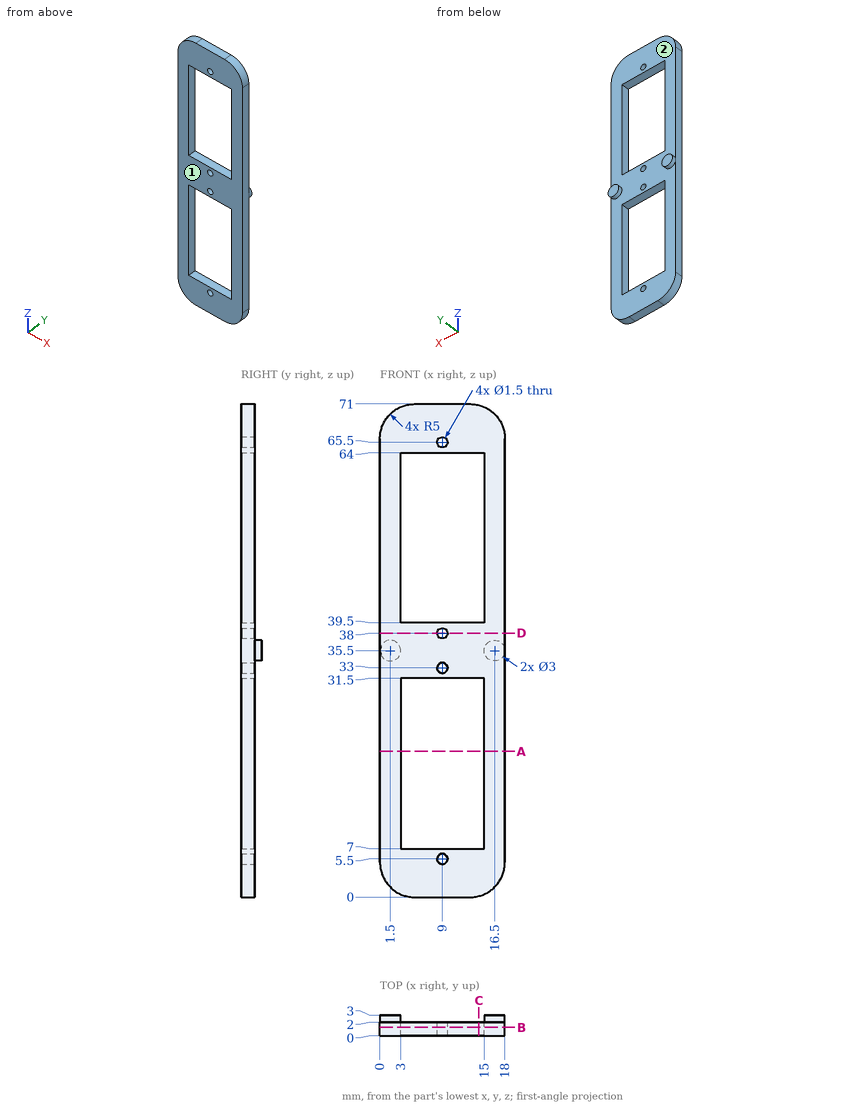
Design review of the part shown in the three views and the two pictorial views. Dimensions are in mm from the part's minimum x, y and z. A direction names the side the tool comes from. Round coordinates to 2 decimals unless told otherwise and drop trailing zeros. Write each loop counter-clockwise with the first axis right and the second up, starting at its lowest first coordinate (ties: lowest second). Pieces come first, ordered by that corner, then holes. Notation, with made-up numbers: M 5,79.25 L 24,79.25 A22 ccw 24,99.25 Z; hole C 76,78 d6. An arc over 180 degrees is marked long. Use a Markdown table: item, result. Add a question column.
Q1. Machinability: for the marked faces 1 and 2, which of the approach directions +Z, -Z, +X, -X, +Y, -Y give a long, thin tool a straight path to every point of the face, cutting with its end or side? Answer none if there is none.
Q2. We need section D-D, the plane z = 38. State the section outline as (x, y) points.
Q3. To check wall thickness, follow line 1 (Z direction, x = 5.5, y = 0.4); line 2 (X direction, y = 0.55, z = 27.5); line 3 (X direction, y = 0.9, z = 5.5). State the ranges of each line that lie inside material, in increasing order.
Q4. We need section B-B, the plane y = 1.25. State the section outline as (x, z) points.
Q5. We need section A-A, the plane z = 21. State the section outline as (x, y) points, plus the area to 3 significant figures.
Q6. Insertion check: pin 1 (0.6 mm diameter, centred on x = 6.5, y = 1, fed in from -Z); pin 2 (6 mm diameter, centred on x = 8, z = 51.5, fed in from -Y). Each pin has a flat end and moves straight along its axis. Give the tip position at first contact, or say it passes through.
Q7. We need section C-C, the plane x = 14.25. State the section outline as (y, z) points.
Findings below:
| question | item | result |
|---|---|---|
| 1 | face 1 | +Z, -Z, +X, -X, -Y |
| 1 | face 2 | +Y |
| 2 | outline | M 0,0 L 8.25,0 L 8.25,2 L 0,2 Z; M 9.75,0 L 18,0 L 18,2 L 9.75,2 Z |
| 3 | line 1 | z = 0 to 7, 31.5 to 39.5, 64 to 71 |
| 3 | line 2 | x = 0 to 3, 15 to 18 |
| 3 | line 3 | x = 0 to 8.25, 9.75 to 18 |
| 4 | outline | M 0,5 A5 ccw 5,0 L 13,0 A5 ccw 18,5 L 18,66 A5 ccw 13,71 L 5,71 A5 ccw 0,66 Z; hole M 3,7 L 15,7 L 15,31.5 L 3,31.5 Z; hole M 3,39.5 L 15,39.5 L 15,64 L 3,64 Z; hole C 9,5.5 d1.5; hole C 9,33 d1.5; hole C 9,38 d1.5; hole C 9,65.5 d1.5 |
| 5 | outline | M 0,0 L 3,0 L 3,2 L 0,2 Z; M 15,0 L 18,0 L 18,2 L 15,2 Z |
| 5 | area | 12.0 mm² |
| 6 | pin 1 | stops at z = 0 |
| 6 | pin 2 | passes through |
| 7 | outline | M 0,0.16 L 2,0.16 L 2,7 L 0,7 Z; M 0,31.5 L 2,31.5 L 2,39.5 L 0,39.5 Z; M 0,64 L 2,64 L 2,70.84 L 0,70.84 Z |
